Input: dimensioned drawing with shaded views. Units: mm. Origin: part minimum x, y, z. A direction names the side the tool comes from. Coordinates: 2 decimals unless noted, no trailing zeros. Loops run counter-clockwise (first coordinate to the right, second up) from the corner with the lowest first, then second, coordinate; pieces in that order, holes last. Notation, with made-up numbers: (-14, -19) - (31, -19) arc R17 cw to (31, 7) - close; hole circle Ø2 at (74.25, 8.25). An arc over 180 degrees is marked (long way). Put each result on its own line as item: value. Start each with the question number.
1) Contact query for flat-ended pins moving along their axis: pin 1 Ø3 at (x, y) = (34, 17.1) entering from -Z; pin 2 Ø3 at (y, z) = (22.5, 16.5) entering from -X; pin 3 Ø2.5 at (y, z) = (17.1, 30) entering from +X. Output: stop coordinate, or through.
2) Section B-B on x = 26.5. Output: boundary loops of the cut face in (y, z), and give its area (3 significant figures).
3) Draft query along X for the marked faces 1, 2, 3 and 4. Return one class per face: +X half, -X half, draft (parallel to the pull), parting line (faces both ways), or undercut.
4) Material intervals for line 1 along Y through (x, z) = (67, 30); line 2 along X through (y, z) = (29, 6); line 3 along X through (y, z) = (13.5, 13), sorted ascending. Write a range as from..to.
5) Section D-D on x = 49. Output: boundary loops of the cut face in (y, z).
6) Section A-A on z = 20. Output: boundary loops of the cut face in (x, y).
7) Section C-C on y = 9.6. Output: boundary loops of the cut face in (x, z).
8) Reachability of the marked faces 5 and 6 from +Z, -Z, +X, -X, +Y, -Y: full face, straight path, thin tool, end or side. Return the list, or none.
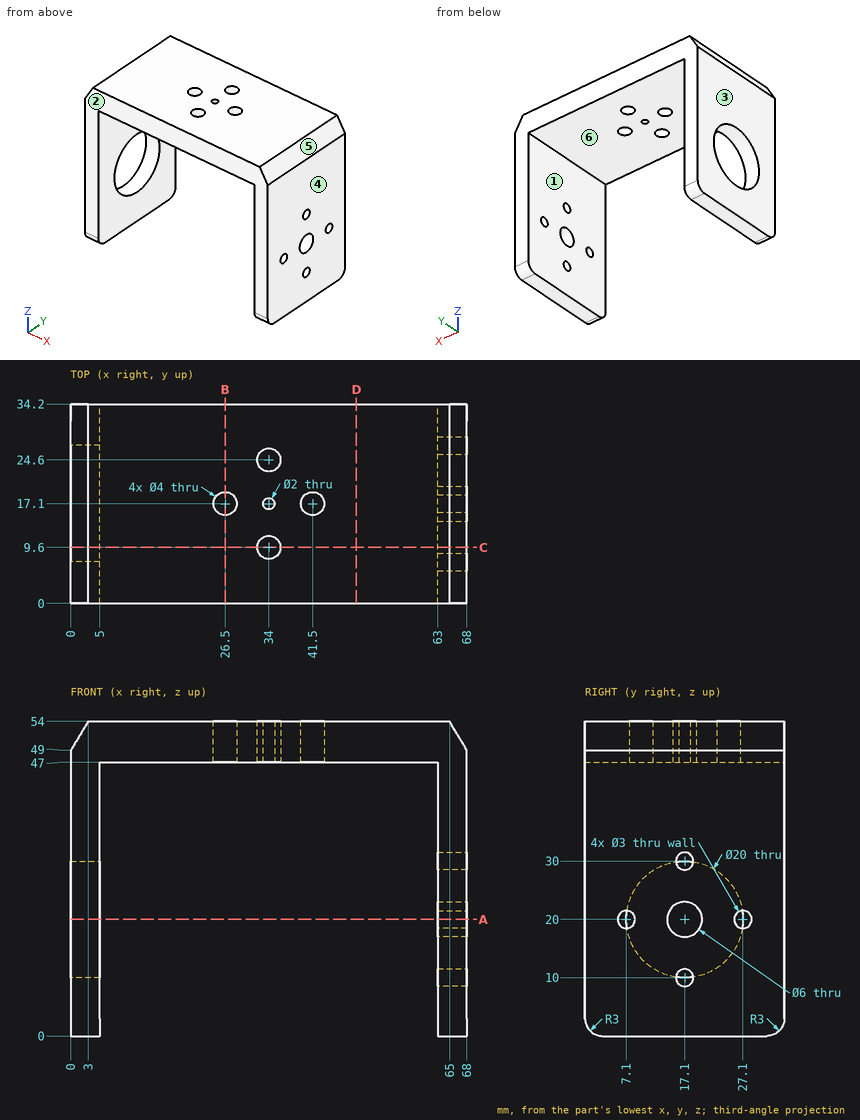
Answer block:
1. pin 1: stops at z = 47
1. pin 2: stops at x = 63
1. pin 3: stops at x = 5
2. outline: (0, 47) - (15.1, 47) - (15.1, 54) - (0, 54) - close; (19.1, 47) - (34.2, 47) - (34.2, 54) - (19.1, 54) - close
2. area: 211 mm²
3. face 1: undercut
3. face 2: draft
3. face 3: -X half
3. face 4: +X half
4. line 1: y = 0..15.6, 18.6..34.2
4. line 2: x = 0..5, 63..68
4. line 3: x = 63..68
5. outline: (0, 47) - (34.2, 47) - (34.2, 54) - (0, 54) - close
6. outline: (0, 0) - (5, 0) - (5, 7.1) - (0, 7.1) - close; (0, 27.1) - (5, 27.1) - (5, 34.2) - (0, 34.2) - close; (63, 0) - (68, 0) - (68, 5.6) - (63, 5.6) - close; (63, 8.6) - (68, 8.6) - (68, 14.1) - (63, 14.1) - close; (63, 20.1) - (68, 20.1) - (68, 25.6) - (63, 25.6) - close; (63, 28.6) - (68, 28.6) - (68, 34.2) - (63, 34.2) - close
7. outline: (0, 0) - (5, 0) - (5, 13.39) - (0, 13.39) - close; (0, 26.61) - (5, 26.61) - (5, 47) - (32, 47) - (32, 54) - (3, 54) - (0, 49) - close; (36, 47) - (63, 47) - (63, 0) - (68, 0) - (68, 49) - (65, 54) - (36, 54) - close
8. face 5: +Z, +X, +Y, -Y
8. face 6: -Z, +Y, -Y
